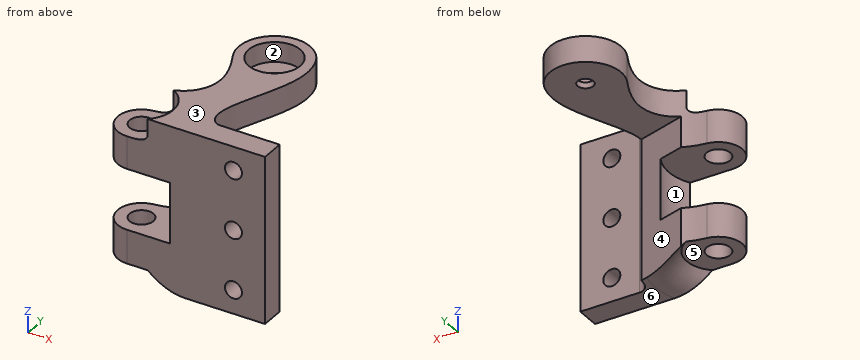
```python
from build123d import *

# Parameters (mm, degrees)
SKETCH1_R           = 6.5
SKETCH1_R_2         = 3.000000000000001
SKETCH1_R_3         = 2.000000000000001
BOSS_EXTRUDE1_DEPTH = 21
CUT_EXTRUDE1_START  = -35.5
CUT_EXTRUDE1_DEPTH  = 35.5
CUT_EXTRUDE2_START  = -14.2
CUT_EXTRUDE2_DEPTH  = 15.3
SKETCH4_R           = 2.1500000000000012
SKETCH4_R_2         = 2.149999999999999
CUT_EXTRUDE3_DEPTH  = 15.3
SKETCH6_R           = 6.499999999999999
CUT_EXTRUDE4_DEPTH  = 5
SKETCH7_R           = 8.000000000000002
CUT_EXTRUDE5_DEPTH  = 6
CUT_EXTRUDE6_START  = -4
SKETCH8_R           = 8.000000000000002
CUT_EXTRUDE6_DEPTH  = 4
FILLET1_R           = 10
FILLET3_R           = 2


with BuildPart() as part:
    # Sketch1 → Boss-Extrude1 (new, symmetric)
    # profile 1 of 2: a face of its own
    with BuildSketch(Plane.XY):
        with BuildLine():
            add(Edge.make_bspline(
                [(8.542559375854681, 32.832786492130545), (10.686678203257555, 26.366975375458193), (5.856141786689584, 16.523631312439278), (0.5083868378802346, 2.514637421674764), (4.080331624706952, -3.187e-14), (4.9722311918748305, 5.6e-16)],
                knots=[0, 0, 0, 0, 0.5826135462254243, 0.9212236747100581, 1, 1, 1, 1], degree=3))
            Line((4.9722311918748305, 5.6e-16), (19.97223119187482, -6.1e-16))
            Line((19.97223119187482, -6.1e-16), (20.000000000000004, -6.000000000000001))
            Line((20.000000000000004, -6.000000000000001), (-15, -6.000000000000003))
            ThreePointArc((-15, -6.000000000000003), (-20.98762892620649, -0.38509718520825564), (-15.768606348517892, 5.950566719314891))
            add(Edge.make_bspline(
                [(-7.98954445714796, 25.856670497383014), (-4.906742308970248, 19.912131256682922), (-3.6628937282407366, 12.195881997757215), (-9.793673492034818, 6.722320325665471), (-15.768606348517892, 5.950566719314891)],
                knots=[0, 0, 0, 0, 0.5365412355207451, 1, 1, 1, 1], degree=3))
            ThreePointArc((-7.98954445714796, 25.856670497383014), (-3.4990005670363873, 38.29198378145294), (8.542559375854681, 32.832786492130545))
        make_face()
        with Locations((1.388e-14, 30)):
            Circle(SKETCH1_R, mode=Mode.SUBTRACT)
        with Locations(Location((-15, 0, 0), (0, 0, 180))):
            Circle(SKETCH1_R_2, mode=Mode.SUBTRACT)
    # profile 2 of 2: a face of its own
    with BuildSketch(Plane.XY):
        with Locations((1.388e-14, 30)):
            Circle(SKETCH1_R)
        with Locations(Location((1.388e-14, 30, 0), (0, 0, 180))):
            Circle(SKETCH1_R_3, mode=Mode.SUBTRACT)
    extrude(amount=BOSS_EXTRUDE1_DEPTH, both=True)

    # Sketch2 → Cut-Extrude1 (cut)
    with BuildSketch(Plane(origin=(0, 0, -21), x_dir=(-1, 0, 0), z_dir=(0, 0, -1)).offset(CUT_EXTRUDE1_START)):
        with BuildLine():
            Line((10.231277065568076, 7.523716250881215), (-2.057381883744481, 3.999999999999989))
            add(Edge.make_bspline(
                [(-8.542559375854681, 32.832786492130545), (-10.686678203257555, 26.366975375458193), (-6.407471523281442, 17.647094178971816), (-2.0529735437800074, 6.524226588369356), (-2.057381883744481, 3.999999999999989)],
                knots=[0, 0, 0, 0, 0.5826135462254243, 0.8160804851922084, 0.8160804851922084, 0.8160804851922084, 0.8160804851922084], degree=3))
            ThreePointArc((-8.542559375854681, 32.832786492130545), (3.499000567036403, 38.29198378145297), (7.98954445714796, 25.856670497383014))
            add(Edge.make_bspline(
                [(10.231277065568076, 7.523716250881215), (7.863619154783306, 8.719037669732709), (3.881869806613929, 13.55430618913155), (4.906742308970248, 19.912131256682922), (7.98954445714796, 25.856670497383014)],
                knots=[0.17604721488266967, 0.17604721488266967, 0.17604721488266967, 0.17604721488266967, 0.46345876447925494, 1, 1, 1, 1], degree=3))
        make_face()
    extrude(amount=CUT_EXTRUDE1_DEPTH, mode=Mode.SUBTRACT)

    # Sketch3 → Cut-Extrude2 (cut)
    with BuildSketch(Plane.XY.offset(21).offset(CUT_EXTRUDE2_START)):
        with BuildLine():
            Line((-15.000000000000002, -6.000000000000002), (-4.0341439002693456, -6.000000000000003))
            ThreePointArc((-4.0341439002693456, -6.000000000000003), (-2.748923532280786, 2.482161433528555), (-7.234360367683872, 9.795143750910501))
            add(Edge.make_bspline(
                [(-7.234360367683872, 9.795143750910501), (-8.872569061817323, 7.931489713842532), (-11.533359351024282, 6.497613392911335), (-15.768606348517892, 5.950566719314891)],
                knots=[0.6714837826850107, 0.6714837826850107, 0.6714837826850107, 0.6714837826850107, 1, 1, 1, 1], degree=3))
            ThreePointArc((-15.768606348517892, 5.950566719314891), (-20.98762892620649, -0.3850971852082583), (-15.000000000000002, -6.000000000000002))
        make_face()
    extrude(amount=-CUT_EXTRUDE2_DEPTH, mode=Mode.SUBTRACT)

    # Sketch4 → Cut-Extrude3 (cut)
    with BuildSketch(Plane(origin=(0, 0, 0), x_dir=(1, 1.3e-16, 0), z_dir=(-1.3e-16, 1, 0))):
        with Locations(Location((12, 0, 0), (0, 0, 180))):
            Circle(SKETCH4_R)
        with Locations(Location((11.999999999999996, 15, 0), (0, 0, 180))):
            Circle(SKETCH4_R_2)
        with Locations(Location((11.999999999999996, -15, 0), (0, 0, 180))):
            Circle(SKETCH4_R_2)
    extrude(amount=-CUT_EXTRUDE3_DEPTH, mode=Mode.SUBTRACT)

    # Sketch6 → Cut-Extrude4 (cut)
    with BuildSketch(Plane.XY.offset(21)):
        with Locations((1.388e-14, 30)):
            Circle(SKETCH6_R)
    extrude(amount=-CUT_EXTRUDE4_DEPTH, mode=Mode.SUBTRACT)

    # Sketch7 → Cut-Extrude5 (cut)
    with BuildSketch(Plane.XY.offset(21)):
        with Locations((-15, 0)):
            Circle(SKETCH7_R)
    extrude(amount=-CUT_EXTRUDE5_DEPTH, mode=Mode.SUBTRACT)

    # Sketch8 → Cut-Extrude6 (cut)
    with BuildSketch(Plane(origin=(0, 0, -21), x_dir=(-1, 0, 0), z_dir=(0, 0, -1)).offset(CUT_EXTRUDE6_START)):
        with Locations((15, 0)):
            Circle(SKETCH8_R)
    extrude(amount=CUT_EXTRUDE6_DEPTH, mode=Mode.SUBTRACT)

    # Fillet1
    # the kernel refuses this fillet: 10 mm, written as the material it takes off along each edge
    with BuildSketch(Plane(origin=(-15, 0, -21), x_dir=(-0.9934899400699477, -0.11391987965149795, 0), z_dir=(0.11391987965149795, -0.9934899400699477, 0))) as fillet1_piece_1:
        with BuildLine():
            CenterArc((16.000000000000007, -10.000000000000002), FILLET1_R, 90, 53.13010235415598)
            Line((8.000000000000004, -4), (8.000000000000004, 0))
            Line((8.000000000000004, 0), (16.000000000000007, 0))
        make_face()
    revolve(axis=Axis((-15, 0, -21), (0, 0, -1)), revolution_arc=359.6400000000001, mode=Mode.SUBTRACT)

    # Fillet3
    fillet3_edges = [part.edges().sort_by_distance(p)[0] for p in [
        (-7.0549828149653875, 0.9363236243440207, 15),
    ]]
    fillet(fillet3_edges, radius=FILLET3_R)


solid = part.part
```
Model file for the job. Use its own axes, mm. Face numbers are marked on the shaded views. A direction names the side the tool comes from. Give positions to 0.01 mm unless a question says otherwise; leave off trailing zeros. Loops run counter-clockwise (first coordinate to the right, second up) from the corner with the lowest first, then second, coordinate; pieces in that order, holes last. Notation, with made-up numbers: (10.25, 66) -> (60.25, 66) arc R16 cw to (60.25, 73) -> close; hole circle Ø10 at (-1, 46). An arc over 180 degrees is marked (long way). Write each question's results on one line, items separated by ' | '.
(1) Tool access for the marked faces 1, 2 and 3: list every direction of +Z, -Z, +X, -X, +Y, -Y with a clear straight run to the whole face (end or side of a thin tool).
Geometry results:
face 1: -X | face 2: +Z | face 3: +Z, +X, -X, +Y, -Y
(2) Pull direction Y, two halves, no side cores. Call the marked faces 4, 5 and 6: released by +Y, released by -Y, zero draft, split by the parting line, or undercut.
Geometry results:
face 4: released by +Y | face 5: undercut | face 6: zero draft
(3) Flat gauge pins, fed straight in: pin 1 Ø14.5 at (x, y) = (-11, -2.5) entering from -Z; pin 2 Ø11 at (x, y) = (-7.5, 2) entering from -Z; pin 3 Ø2 at (x, z) = (-9, -8.5) entering from +Y. Where does each tip first touch, or does it go through?
Geometry results:
pin 1: stops at z = -20.15 | pin 2: stops at z = -20.62 | pin 3: stops at y = 7.46
(4) Cut at A-A on x = 13.5. List the corners of the cut face in (y, z).
Geometry results:
outline: (-6, -21) -> (0, -21) -> (0, -16.54) -> (-6, -16.54) -> close; (-6, -13.46) -> (0, -13.46) -> (0, -1.54) -> (-6, -1.54) -> close; (-6, 1.54) -> (0, 1.54) -> (0, 13.46) -> (-6, 13.46) -> close; (-6, 16.54) -> (0, 16.54) -> (0, 21) -> (-6, 21) -> close
(5) Cut at B-B on y = 35.5. List the corners of the cut face in (x, z), and give its area (3 significant figures).
Geometry results:
outline: (-7.12, 14.5) -> (7.12, 14.5) -> (7.12, 21) -> (3.46, 21) -> (3.46, 16) -> (-3.46, 16) -> (-3.46, 21) -> (-7.12, 21) -> close | area: 58.0 mm²
(6) Cut at C-C on z = -14. Give the number of separate pieces and of enclosed holes in the cut face, and give its area (3 significant figures).
Geometry results:
separate pieces: 2 | enclosed holes: 1 | area: 320 mm²
(7) Probe line 1 along Z through (x, y) = (12, -4); line 2 along Y through (x, z) = (0, 19); line 3 along Z through (x, y) = (-14, 3). List the from-to ranges inside material, lowest first.
Geometry results:
line 1: z = -21 to -17.15, -12.85 to -2.15, 2.15 to 12.85, 17.15 to 21 | line 2: y = -6 to 23.5, 36.5 to 39 | line 3: z = -17 to -8.5, 6.8 to 15
